Model file for the job. Use its own axes, mm. A direction names the side the tool comes from. Coordinates: 2 decimals unless noted, no trailing zeros. Order: outer loops, then holes, each group sorted by start corner. A loop starts at its lowest first (then second) coordinate and runs counter-clockwise, first axis right, second up. Notation, with made-up numbers: M 37.5,71 L 94.5,71 A14 cw 94.5,75 Z; hole C -36,-26.75 d5. An arc over 180 degrees is marked long. Return JSON: item names as keys, results as strings.
```python
from build123d import *

# Parameters (mm, degrees)
F0_R     = 7.5
F1_DEPTH = 0.8
F3_R     = 3.85
F3_R_2   = 2.85
F4_DEPTH = 6


with BuildPart() as f1:
    # F0 (on Front) → F1 (new body)
    with BuildSketch(Plane.XZ):
        Circle(F0_R)
    extrude(amount=F1_DEPTH)

    # F3 (on face) → F4 (join)
    with BuildSketch(Plane.XZ.offset(0.8)):
        Circle(F3_R)
        Circle(F3_R_2, mode=Mode.SUBTRACT)
    extrude(amount=F4_DEPTH)


solid = f1.part
```
Item 1: Pull direction Z, two halves, no side cores. Call faces 3 (the cylindrical face through (-7.493, -0.394, 0.33)), 4 (the flat face through (0, 0, 0)), 5 (the flat face through (0, -0.8, 0)), 6 (the cylindrical face through (-2.262, -3.758, -1.734)): +Z half, -Z half, draft (parallel to the pull), parting line (faces both ways), or undercut.
Check result:
{"face 3": "parting line", "face 4": "draft", "face 5": "undercut", "face 6": "undercut"}
Item 2: Saw through at B-B (y = -3). Write the cut outline in (x, z).
Check result:
{"outline": "C 0,0 d7.7; hole C 0,0 d5.7"}
Item 3: Saw through at D-D (x = 3.25). Write the cut outline in (y, z).
Check result:
{"outline": "M -6.8,-2.06 L -0.8,-2.06 L -0.8,-6.76 L 0,-6.76 L 0,6.76 L -0.8,6.76 L -0.8,2.06 L -6.8,2.06 Z"}
Item 4: Wall check: line 1 (Z direction, x = 0, y = -2.4); line 2 (Y direction, x = 6.25, z = -3.25); line 3 (Z direction, x = -1.75, y = -6). Give the ranges that are in metal, low to high.
Check result:
{"line 1": "z = -3.85 to -2.85, 2.85 to 3.85", "line 2": "y = -0.8 to 0", "line 3": "z = -3.43 to -2.25, 2.25 to 3.43"}
Item 5: Saw through at A-A (x = 0). Write the cut outline in (y, z).
Check result:
{"outline": "M -6.8,-3.85 L -0.8,-3.85 L -0.8,-7.5 L 0,-7.5 L 0,7.5 L -0.8,7.5 L -0.8,3.85 L -6.8,3.85 L -6.8,2.85 L -0.8,2.85 L -0.8,-2.85 L -6.8,-2.85 Z"}
Item 6: Saw through at C-C (z = 0). Write the cut outline in (x, y), and give its area (3 significant figures).
Check result:
{"outline": "M -7.5,-0.8 L -3.85,-0.8 L -3.85,-6.8 L -2.85,-6.8 L -2.85,-0.8 L 2.85,-0.8 L 2.85,-6.8 L 3.85,-6.8 L 3.85,-0.8 L 7.5,-0.8 L 7.5,0 L -7.5,0 Z", "area": "24.0 mm2"}
Item 7: Drop flat-ended pins along their axis: pin 1 Ø3 at (y, z) = (-3.5, -2) entering from -X; pin 2 Ø3 at (y, z) = (-6, -3.5) entering from -X; pin 3 Ø2 at (x, y) = (5, -5) entering from -Z. Give the stop position or say it passes through.
Check result:
{"pin 1": "stops at x = -3.82", "pin 2": "stops at x = -3.29", "pin 3": "passes through"}
Item 8: 3-axis set-ups, long thin cutter, end or side, ignore diameter. For faces 1 (the flat face through (1, -6.8, 3)), 2 (the flat face through (3, -0.8, -3)): which of +Z, -Z, +X, -X, +Y, -Y reach the whole face in a straight line?
Check result:
{"face 1": "+Z, -Z, +X, -X, -Y", "face 2": "-Y"}
